Source: CAD feature listing. Evaluate the final solid. Frame: model axes, mm. A direction names the side the tool comes from. Coordinates: 2 decimals unless noted, no trailing zeros. Loops run counter-clockwise (first coordinate to the right, second up) from the corner with the lowest first, then second, coordinate; pieces in that order, holes last. Notation, with made-up numbers: (78, 89.25) -> (98, 89.25) arc R19 ccw to (98, 124.25) -> close; hole circle Ø8 at (89.25, 78). An arc over 180 degrees is marked (long way). Answer as CSV lines item,"result".
from build123d import *

# Parameters (mm, degrees)
F0_W     = 86.909074
F0_H     = 24
F1_DEPTH = 10
F2_W     = 10
F2_H     = 24
F3_DEPTH = 95
F4_W     = 24
F4_H     = 10
F5_DEPTH = 76.909075
F6_W     = 60
F6_H     = 10
F7_DEPTH = 24


with BuildPart() as f1:
    # F0 (on Top) → F1 (new body)
    with BuildSketch(Plane.XY):
        Rectangle(F0_W, F0_H)
    extrude(amount=F1_DEPTH)

    # F2 (on face) → F3 (join)
    with BuildSketch(Plane.XY.offset(10)):
        with Locations((38.454537, 0)):
            Rectangle(F2_W, F2_H)
    extrude(amount=F3_DEPTH)

    # F4 (on face) → F5 (join, through all)
    with BuildSketch(Plane(origin=(33.454537, 0, 0), x_dir=(0, -1, 0), z_dir=(-1, 0, 0))):
        with Locations((0, 17)):
            Rectangle(F4_W, F4_H)
    extrude(amount=F5_DEPTH)

    # F6 (on face) → F7 (join, through all)
    with BuildSketch(Plane.XZ.offset(12)):
        Polygon((-26.545463, 92), (-26.545463, 22), (-16.545463, 22), (-16.545463, 82), (33.454537, 82), (33.454537, 92), align=None)
        with Locations((3.454537, 100)):
            Rectangle(F6_W, F6_H)
    extrude(amount=-F7_DEPTH)


solid = f1.part
(1) Cut plane A-A (x = -30). Return the cut outline in (y, z).
Computed values:
outline,"(-12, 0) -> (12, 0) -> (12, 10) -> (-12, 10) -> close; (-12, 12) -> (12, 12) -> (12, 22) -> (-12, 22) -> close"
(2) Pin query (flat end, axial travel): pin 1 Ø0.9 at (y, z) = (-5.5, 94) entering from -X; pin 2 Ø12 at (y, z) = (-6, 54) entering from -X. Return the tip coordinate at first contact, or that it passes through.
Computed values:
pin 1,"x = 33.45"
pin 2,"x = -26.55"
(3) Material intervals for L1, parallel to Z at x = 1.5, y = 1; L2, parallel to Z at x = -18, y = 6.5; L3, parallel to X at y = -0.75, z = 40.5, sorted ascending. Write a range as [from, to].
Computed values:
L1,"[0, 10], [12, 22], [82, 92], [95, 105]"
L2,"[0, 10], [12, 92], [95, 105]"
L3,"[-26.55, -16.55], [33.45, 43.45]"
(4) Cut plane D-D (y = -2). Return the cut outline in (x, z).
Computed values:
outline,"(-43.45, 0) -> (43.45, 0) -> (43.45, 105) -> (-26.55, 105) -> (-26.55, 95) -> (33.45, 95) -> (33.45, 92) -> (-26.55, 92) -> (-26.55, 22) -> (-43.45, 22) -> (-43.45, 12) -> (33.45, 12) -> (33.45, 10) -> (-43.45, 10) -> close; hole (-16.55, 22) -> (33.45, 22) -> (33.45, 82) -> (-16.55, 82) -> close"
(5) Access query for faces 1 (the flat face through (-26.545, 0, 57)), 2 (the flat face through (-4, 0, 12)), 3 (the flat face through (9, 0, 22)). Directions: +Z, -Z, +X, -X, +Y, -Y. A direction counts if a zero-diameter tool reaches every point of the face in a straight line with its end or side. Return the directions, or none.
Computed values:
face 1,"+Z, -X, +Y, -Y"
face 2,"-X, +Y, -Y"
face 3,"+Y, -Y"
(6) Draft query along X for faces 4 (the flat face through (33.455, 0, 93)), 5 (the flat face through (-35, 0, 22)), 6 (the flat face through (8, 0, 82)). Return one class per face: released by +X, released by -X, zero draft, split by the parting line, or undercut.
Computed values:
face 4,"released by -X"
face 5,"zero draft"
face 6,"undercut"
(7) Cut plane B-B (z = 56). Return the cut outline in (x, y).
Computed values:
outline,"(-26.55, -12) -> (-16.55, -12) -> (-16.55, 12) -> (-26.55, 12) -> close; (33.45, -12) -> (43.45, -12) -> (43.45, 12) -> (33.45, 12) -> close"
(8) Cut plane C-C (x = 2.5). Return the cut outline in (y, z), then the cut area to 3 significant figures.
Computed values:
outline,"(-12, 0) -> (12, 0) -> (12, 10) -> (-12, 10) -> close; (-12, 12) -> (12, 12) -> (12, 22) -> (-12, 22) -> close; (-12, 82) -> (12, 82) -> (12, 92) -> (-12, 92) -> close; (-12, 95) -> (12, 95) -> (12, 105) -> (-12, 105) -> close"
area,"960 mm^2"
